Autodesk Inventor part; units mm, degrees
ref_plane "YZ Plane" through (0, 0, 0) normal (1, 0, 0) x (0, 1, 0)
ref_plane "XZ Plane" through (0, 0, 0) normal (0, 1, 0) x (-1, 0, 0)
ref_plane "XY Plane" through (0, 0, 0) normal (0, 0, 1) x (1, 0, 0)
sketch "Эскиз1" plane through (0, 0, 0) normal (0, 1, 0) x (-1, 0, 0)
  circle A0 centre (0, 0) radius 12.5 construction
  circle A1 centre (0, 0) radius 8.5 construction
  circle A2 centre (6.0104, 6.0104) radius 1.5
  circle A3 centre (-6.0104, -6.0104) radius 1.5
  circle A4 centre (0, 0) radius 4
  line L0 (27.5, 25) -> (-12.5, 25)
  line L1 (-12.5, 25) -> (-12.5, -25)
  line L2 (-12.5, -25) -> (27.5, -25)
  line L3 (27.5, -25) -> (27.5, 25)
  line L4 (8.8388, -8.8388) -> (-8.8388, 8.8388) construction
  line L5 (-8.8388, -8.8388) -> (8.8388, 8.8388) construction
  circle A5 centre (6.0104, -6.0104) radius 1.5
  circle A6 centre (-6.0104, 6.0104) radius 1.5
  point P0 (7.5, 25)
  point P1 (7.5, -25)
  dimension "d0" = 25
  dimension "d1" = 17
  dimension "d2" = 3
  dimension "d3" = 3
  dimension "d4" = 8
  dimension "d5" = 40
  dimension "d6" = 50
  dimension "d7" = 25
  dimension "d26" = 25
  dimension "d31" = 45
  dimension "d32" = 90
  dimension "d33" = 3
  dimension "d34" = 3
extrude "Выдавливание1" add sketch "Эскиз1" along normal blind 2.5
sketch "Эскиз2" plane through (0, 0, 0) normal (0, -1, 0) x (1, 0, 0)
  circle A0 centre (0, 0) radius 13
  line L0 (12.5, 25) -> (12.5, -25)
  line L1 (-27.5, 25) -> (12.5, 25)
  line L2 (-27.5, -25) -> (-27.5, 25)
  line L3 (12.5, -25) -> (-27.5, -25)
  circle A1 centre (-6.0104, 6.0104) radius 1.5
  circle A2 centre (6.0104, -6.0104) radius 1.5
  circle A3 centre (0, 0) radius 4
  point P0 (12.5, -3.5707)
  point P1 (12.5, 3.5707)
  dimension "d10" = 26
extrude "Выдавливание2" add sketch "Эскиз2" along normal blind 7.5 contours A0 L0 L3 L2 L1
fillet "Сопряжение1" radius 2 4 edges at (-7.5, -7.5, -25) (-7.5, 2.5, -25) (-7.5, -7.5, 25) (-7.5, 2.5, 25)
sketch "Эскиз4" plane through (-27.5, -5.5, -25) normal (-1, 0, 0) x (0, 0, 1)
  arc A0 (50, 6) -> (48, 8) centre (48, 6) ccw
  line L0 (2, 8) -> (48, 8)
  arc A1 (2, 8) -> (0, 6) centre (2, 6) ccw
  line L1 (0, 0) -> (0, 6)
  arc A2 (0, 0) -> (2, -2) centre (2, 0) ccw
  line L2 (48, -2) -> (2, -2)
  arc A3 (48, -2) -> (50, 0) centre (48, 0) ccw
  line L3 (50, 0) -> (50, 6)
  circle A4 centre (42, 3) radius 1.65
  circle A5 centre (8, 3) radius 1.65
  point P0 (25, 5.5)
  point P1 (50, 3)
  dimension "d21" = 3.3
  dimension "d22" = 3.3
  dimension "d41" = 5
  dimension "d42" = 34
  dimension "d43" = 8
  dimension "d44" = 5
extrude "Выдавливание4" cut sketch "Эскиз4" against normal through all contours A4 | A5
chamfer "Фаска1" distance 2 angle 45 4 edges at (-4.5104, 2.5, 6.0104) (7.5104, 2.5, -6.0104) (-4.5104, 2.5, -6.0104) (7.5104, 2.5, 6.0104)
sketch "Эскиз5" plane through (0, -7.5, 0) normal (0, -1, 0) x (1, 0, 0)
  line L0 (-27.5, 23) -> (12.5, 23)
  line L1 (-27.5, 23) -> (-27.5, -23)
  line L2 (12.5, -23) -> (-27.5, -23)
  line L3 (12.5, -23) -> (12.5, -3.5707)
  arc A0 (12.5, 3.5707) -> (12.5, -3.5707) centre (0, 0) ccw
  line L4 (12.5, 3.5707) -> (12.5, 23)
  line L5 (-27.5, -18.65) -> (12.5, -18.65)
  line L6 (-27.5, -15.35) -> (12.5, -15.35)
  line L7 (12.5, -18.65) -> (12.5, -15.35)
  line L8 (12.5, -17) -> (-27.5, -17) construction
  line L9 (9, -14.1) -> (6, -14.1)
  line L10 (6, -14.1) -> (6, -19.9)
  line L11 (6, -19.9) -> (9, -19.9)
  line L12 (9, -19.9) -> (9, -14.1)
  line L13 (9, -14.1) -> (6, -19.9) construction
  line L14 (6, -14.1) -> (9, -19.9) construction
  circle A1 centre (0, 0) radius 4
  line L15 (0, 0) -> (12.5, 0) construction
  line L16 (12.5, 3.5707) -> (12.5, -3.5707)
  line L17 (-7.5, -23) -> (-7.5, 23) construction
  line L18 (9, 14.1) -> (6, 14.1)
  line L19 (6, 14.1) -> (6, 19.9)
  line L20 (6, 19.9) -> (9, 19.9)
  line L21 (9, 19.9) -> (9, 14.1)
  line L22 (9, 14.1) -> (6, 19.9) construction
  line L23 (6, 14.1) -> (9, 19.9) construction
  line L24 (-24, -14.1) -> (-21, -14.1)
  line L25 (-21, -14.1) -> (-21, -19.9)
  line L26 (-21, -19.9) -> (-24, -19.9)
  line L27 (-24, -19.9) -> (-24, -14.1)
  line L28 (-24, -14.1) -> (-21, -19.9) construction
  line L29 (-21, -14.1) -> (-24, -19.9) construction
  line L30 (-21, 14.1) -> (-21, 19.9)
  line L31 (-21, 19.9) -> (-24, 19.9)
  line L32 (-24, 14.1) -> (-21, 14.1)
  line L33 (-24, 19.9) -> (-24, 14.1)
  line L34 (-24, 14.1) -> (-21, 19.9) construction
  line L35 (-21, 14.1) -> (-24, 19.9) construction
  point P0 (7.5, -17)
  point P1 (12.5, -13.2854)
  point P2 (7.5, 17)
  point P3 (-22.5, -17)
  point P4 (-22.5, 17)
  dimension "d35" = 3
  dimension "d36" = 5.8
  dimension "d38" = 5
extrude "Выдавливание5" cut sketch "Эскиз5" against normal blind 8.5 contours L27 L24 L25 L6 | L6 L25 L5 L27 | L5 L25 L26 L27 | L10 L9 L12 L6 | L6 L12 L5 L10 | L5 L12 L11 L10 | L18 L19 L20 L21 | L32 L33 L31 L30
equation "\"d22\" = d21"
properties part number "motoramma"
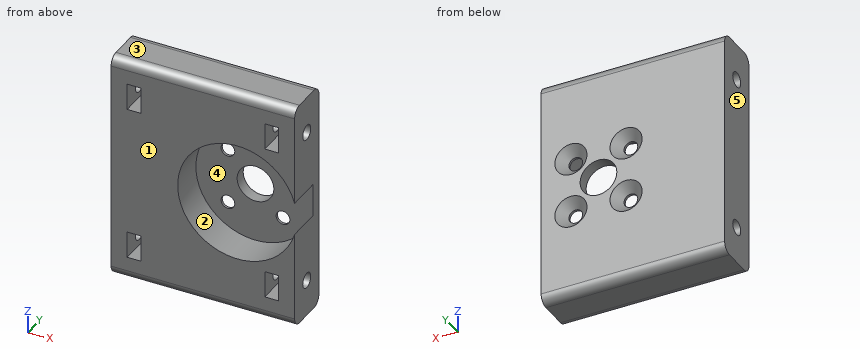
Could you check a few things on this model? Use its own coordinates, in mm. Face numbers are marked on the shaded views. A direction names the side the tool comes from. Coordinates: 2 decimals unless noted, no trailing zeros. Order: outer loops, then holes, each group sorted by start corner. A loop starts at its lowest first (then second) coordinate and runs counter-clockwise, first axis right, second up. Notation, with made-up numbers: M 79.5,52 L 107.5,52 A20 ccw 107.5,68 Z; hole C 6.5,-32 d7. An arc over 180 degrees is marked long. Use a Markdown table: item, result. Add a question column.
Q1. I'm going to push flat-ended pins straight in: pin 1 (0.9 mm diameter, centred on x = -22, z = -16, fed in from -Y); pin 2 (3.5 mm diameter, centred on x = -6.01, z = -6.01, fed in from -Y). Where does each tip first touch, or does it pass through?
Q2. If I drill on L1, parallel to X at y = -6.25, z = 19.5; L2, parallel to Y at x = -24.7, z = 17; L3, parallel to Z at x = -1, y = -2.75, over which ranges is the centre line in solid material (lowest first)?
Q3. I want a section at B-B on z = 0. List the corners of the cut face in (x, y) for me, then the cut area to 3 significant figures.
Q4. I want a section at A-A on x = 0. List the corners of the cut face in (y, z) for me, then the cut area to 3 significant figures.
Q5. I want a section at D-D on x = -12. List the corners of the cut face in (y, z) for me.
Q6. Which directions (+Z, -Z, +X, -X, +Y, -Y) give clear straight access to the entire face, cutting with the end or side of a thin tool? Please do the marked faces 4 and 5.
Q7. I want a section at C-C on z = 17. List the corners of the cut face in (x, y) for me.
Q8. We'd pull the mould along Z, two halves only. Please class the marked faces 1, 2 and 3: pulls with the +Z half, pulls with the -Z half, needs draft (parallel to the pull), parting line crosses it, or undercut.
Checked values:
| question | item | result |
|---|---|---|
| 1 | pin 1 | y = 1 |
| 1 | pin 2 | y = 0 |
| 2 | L1 | -27.5 to -24, -21 to 6, 9 to 12.5 |
| 2 | L2 | -7.5 to -4.15, -0.85 to 2.5 |
| 2 | L3 | -25 to -18.63, -15.37 to -12.96, 12.96 to 15.37, 18.63 to 25 |
| 3 | outline | M -27.5,-7.5 L -13,-7.5 L -13,0 L -4,0 L -4,2.5 L -27.5,2.5 Z; M 4,0 L 12.5,0 L 12.5,2.5 L 4,2.5 Z |
| 3 | area | 189 mm² |
| 4 | outline | M -7.5,-23 A2 ccw -5.5,-25 L 0.5,-25 A2 ccw 2.5,-23 L 2.5,-4 L 0,-4 L 0,-13 L -7.5,-13 Z; M -7.5,13 L 0,13 L 0,4 L 2.5,4 L 2.5,23 A2 ccw 0.5,25 L -5.5,25 A2 ccw -7.5,23 Z; hole C -2.5,-17 d3.3; hole C -2.5,17 d3.3 |
| 4 | area | 264 mm² |
| 5 | outline | M -7.5,-23 A2 ccw -5.5,-25 L 0.5,-25 A2 ccw 2.5,-23 L 2.5,23 A2 ccw 0.5,25 L -5.5,25 A2 ccw -7.5,23 L -7.5,5 L 0,5 L 0,-5 L -7.5,-5 Z; hole C -2.5,-17 d3.3; hole C -2.5,17 d3.3 |
| 6 | face 4 | -Y |
| 6 | face 5 | +Z, -Z, -X, +Y, -Y |
| 7 | outline | M -27.5,-7.5 L -24,-7.5 L -24,-4.15 L -27.5,-4.15 Z; M -27.5,-0.85 L -24,-0.85 L -24,1 L -21,1 L -21,-0.85 L 6,-0.85 L 6,1 L 9,1 L 9,-0.85 L 12.5,-0.85 L 12.5,2.5 L -27.5,2.5 Z; M -21,-7.5 L 6,-7.5 L 6,-4.15 L -21,-4.15 Z; M 9,-7.5 L 12.5,-7.5 L 12.5,-4.15 L 9,-4.15 Z |
| 8 | face 1 | needs draft |
| 8 | face 2 | undercut |
| 8 | face 3 | pulls with the +Z half |
